from build123d import *

# Parameters (mm, degrees)
F1_DEPTH  = 38.1
F2_W      = 50.8
F2_H      = 3.175
F3_DEPTH  = 6.35
F5_DEPTH  = 25.4
F6_W      = 44.45
F6_H      = 6.35
F7_DEPTH  = 6.35
F9_DEPTH  = 25.4
F10_R     = 4.1275
F11_DEPTH = 127
F13_DEPTH = 127


# Not quite as in the source:
# - a feature names something its author has since deleted; it is built from what else it names


with BuildPart() as f1:
    # F0 (on Top) → F1 (new body)
    with BuildSketch(Plane.XY):
        Polygon((43.9940905122, -25.4), (50.8, 0), (43.9940905122, 25.4), (25.4, 43.9940905122), (0, 50.8), (-25.4, 43.9940905122), (-43.9940905122, 25.4), (-50.8, 0), (0, 0), (0, -50.8), (25.4, -43.9940905122), align=None)
    extrude(amount=F1_DEPTH)

    # F2 (on face) → F3 (join)
    with BuildSketch(Plane.XZ):
        with Locations((-25.4, 20.6375)):
            Rectangle(F2_W, F2_H)
        with Locations((-25.4, 17.4625)):
            Rectangle(F2_W, F2_H)
    extrude(amount=F3_DEPTH)

    # F4 (on face) → F5 (cut)
    with BuildSketch(Plane.XY.offset(22.225)):
        Polygon((-49.0985226281, -6.35), (-50.8, 0), (-50.8, -6.35), align=None)
    extrude(amount=-F5_DEPTH, mode=Mode.SUBTRACT)

    # F6 (on face) → F7 (join)
    with BuildSketch(Plane(origin=(0, 0, 0), x_dir=(0, -1, 0), z_dir=(-1, 0, 0))):
        with Locations((28.575, 19.05)):
            Rectangle(F6_W, F6_H)
    extrude(amount=F7_DEPTH)

    # F8 (on face) → F9 (cut)
    with BuildSketch(Plane.XY.offset(22.225)):
        Polygon((-6.35, -50.8), (0, -50.8), (-6.35, -49.0985226281), align=None)
    extrude(amount=-F9_DEPTH, mode=Mode.SUBTRACT)

    # F10 (on face) → F11 (cut)
    with BuildSketch(Plane.XY.offset(38.1)):
        Circle(F10_R)
    extrude(amount=-F11_DEPTH, mode=Mode.SUBTRACT)

    # F12 (on face) → F13 (cut)
    with BuildSketch(Plane.XY.offset(38.1)):
        with BuildLine():
            ThreePointArc((-4.1275, 0), (-3.8133127704, 1.5795258671), (-2.9185832393, 2.9185832393))
            Line((-2.9185832393, 2.9185832393), (-5.8371664787, 0))
            Line((-5.8371664787, 0), (-4.1275, 0))
        make_face()
        with BuildLine():
            ThreePointArc((4.1275, 0), (1.5795258671, 3.8133127704), (-2.9185832393, 2.9185832393))
            ThreePointArc((-2.9185832393, 2.9185832393), (-3.8133127704, 1.5795258671), (-4.1275, 0))
            Line((-4.1275, 0), (-5.8371664787, 0))
            Line((-5.8371664787, 0), (-18.7979032201, -12.9607367414))
            Line((-18.7979032201, -12.9607367414), (-12.9607367414, -18.7979032201))
            Line((-12.9607367414, -18.7979032201), (0, -5.8371664787))
            Line((0, -5.8371664787), (0, -4.1275))
            ThreePointArc((0, -4.1275), (1.5795258671, -3.8133127704), (2.9185832393, -2.9185832393))
            ThreePointArc((2.9185832393, -2.9185832393), (3.8133127704, -1.5795258671), (4.1275, 0))
        make_face()
        with BuildLine():
            Line((0, -5.8371664787), (2.9185832393, -2.9185832393))
            ThreePointArc((2.9185832393, -2.9185832393), (1.5795258671, -3.8133127704), (0, -4.1275))
            Line((0, -4.1275), (0, -5.8371664787))
        make_face()
    extrude(amount=-F13_DEPTH, mode=Mode.SUBTRACT)


solid = f1.part
Input: part model. Units: mm. Frame: model coordinates. A direction names the side the tool comes from. Round coordinates to 2 decimals unless told otherwise and drop trailing zeros. Order: outer loops, then holes, each group sorted by start corner. A loop starts at its lowest first (then second) coordinate and runs counter-clockwise, first axis right, second up. Notation, with made-up numbers: (37.25, -28) - (66.25, -28) arc R15 cw to (66.25, -1) - close; hole circle Ø4 at (31.5, -7.75). An arc over 180 degrees is marked (long way). Use a Markdown table: item, result.
1. Material intervals for probe 1 along Y at (x, z) = (2.5, 34.5); probe 2 along X at (y, z) = (1.5, 2.5); probe 3 along Z at (x, y) = (-5, -13) (3 decimals), sorted ascending.
Evaluation:
| item | result |
|---|---|
| probe 1 | -50.13 to -3.34, 3.28 to 50.13 |
| probe 2 | -50.4 to -4.34, 3.85 to 50.4 |
| probe 3 | 15.875 to 22.225 |
2. Access query for faces 1 (the face through (-28, -3, 15.875)), 2 (the face through (-47.35, 12.88, 18.78)), 3 (the face through (-31, -6.35, 19)), 4 (the face through (-3, -28, 22.225)), 5 (the face through (34.567, -34.827, 18.783)). Directions: +Z, -Z, +X, -X, +Y, -Y. A direction counts if a zero-diameter tool reaches every point of the face in a straight line with its end or side. Return the directions, or none.
Evaluation:
| item | result |
|---|---|
| face 1 | -Z, -X, -Y |
| face 2 | +Z, -Z, -X, +Y |
| face 3 | +Z, -Z, -X, -Y |
| face 4 | +Z, -X, -Y |
| face 5 | +Z, -Z, +X, -Y |
3. Section A-A on x = -21.5. Return the cut outline in (y, z) (3 decimals).
Evaluation:
| item | result |
|---|---|
| outline | (-6.35, 15.875) - (0, 15.875) - (0, 0) - (45.039, 0) - (45.039, 38.1) - (0, 38.1) - (0, 22.225) - (-6.35, 22.225) - close |
4. Section B-B on z = 3. Return the cut outline in (x, y) (1 decimal).
Evaluation:
| item | result |
|---|---|
| outline | (-50.8, 0) - (-5.8, 0) - (-2.9, 2.9) arc R4.1 cw to (2.9, -2.9) - (0, -5.8) - (0, -50.8) - (25.4, -44) - (44, -25.4) - (50.8, 0) - (44, 25.4) - (25.4, 44) - (0, 50.8) - (-25.4, 44) - (-44, 25.4) - close |
5. Section C-C on y = -35. Return the cut outline in (x, z) (3 decimals), then the cut area to 3 significant figures.
Evaluation:
| item | result |
|---|---|
| outline | (-6.35, 15.875) - (0, 15.875) - (0, 0) - (34.394, 0) - (34.394, 38.1) - (0, 38.1) - (0, 22.225) - (-6.35, 22.225) - close |
| area | 1,350 mm^2 |
6. Section D-D on y = 23.5. Return the cut outline in (x, z), then the cut area to 3 significant figures.
Evaluation:
| item | result |
|---|---|
| outline | (-44.5, 0) - (44.5, 0) - (44.5, 38.1) - (-44.5, 38.1) - close |
| area | 3,390 mm^2 |
7. First-contact query: pin 1 (5 mm diameter, centred on x = -4.5, y = -18.5, fed in from -Z) (3 decimals); pin 2 (12 mm diameter, centred on y = -24.5, z = 4.5, fed in from -X); pin 3 (8 mm diameter, centred on y = 18.5, z = 20.5, fed in from +X). Flat tips, straight axial feed; report the tip coordinate or a pass-through.
Evaluation:
| item | result |
|---|---|
| pin 1 | z = 15.875 |
| pin 2 | x = 0 |
| pin 3 | x = 46.91 |
8. Mould query, pull axis Y, two halves, no side actions, for faces 6 (the face through (2.982, 2.854, 19.317)), 7 (the face through (-6.35, -30, 19)), 8 (the face through (-34.567, 34.827, 18.783)). Classes: +Y half, -Y half, draft (parallel to the pull), parting line (faces both ways), or undercut.
Evaluation:
| item | result |
|---|---|
| face 6 | undercut |
| face 7 | draft |
| face 8 | +Y half |
